For this review, take the finished solid that the model builds, in its own axes (mm). Face numbers are marked on the shaded views. A direction names the side the tool comes from. Round coordinates to 2 decimals unless told otherwise and drop trailing zeros. Loops run counter-clockwise (first coordinate to the right, second up) from the corner with the lowest first, then second, coordinate; pieces in that order, holes last. Notation, with made-up numbers: (-9, 55.5) -> (18, 55.5) arc R20 cw to (18, 86.5) -> close; hole circle Ø7 at (-32.5, -5.5). An arc over 180 degrees is marked (long way). Write each question's results on one line, items separated by ' | '.
```python
from build123d import *

# Parameters (mm, degrees)
SKETCH1_W           = 25.4
SKETCH1_H           = 25.4
BOSS_EXTRUDE1_DEPTH = 1.5875
BOSS_EXTRUDE2_DEPTH = 3.302


with BuildPart() as part:
    # Sketch1 → Boss-Extrude1 (new body)
    with BuildSketch(Plane(origin=(0, 0, 0), x_dir=(1, 0, 0), z_dir=(0, 1, 0))):
        with Locations((-11.947275054, 12.711155892)):
            Rectangle(SKETCH1_W, SKETCH1_H)
    extrude(amount=BOSS_EXTRUDE1_DEPTH)

    # Sketch2 → Boss-Extrude2 (add)
    with BuildSketch(Plane(origin=(0, 0, 0), x_dir=(-1, 0, 0), z_dir=(0, -1, 0))):
        Polygon((17.95497638, 12.711155892), (5.939573728, 12.711155892), (4.886075054, 15.759155892), (4.886075054, 25.411155892), (19.008475054, 25.411155892), (19.008475054, 15.759155892), align=None)
    extrude(amount=BOSS_EXTRUDE2_DEPTH)


solid = part.part
```
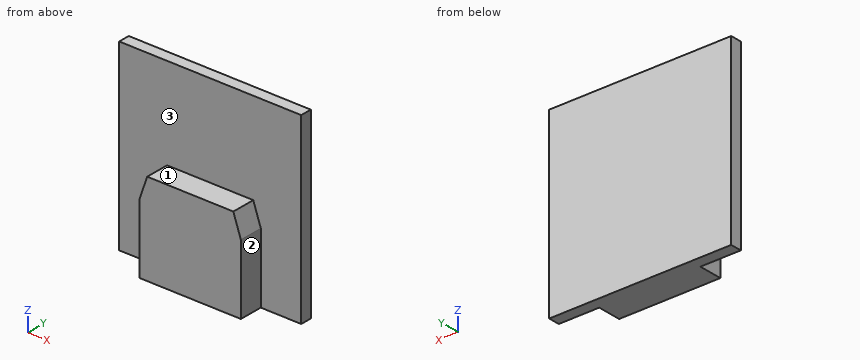
1. To check wall thickness, follow probe 1 along Y at (x, z) = (-2, -20.25); probe 2 along Z at (x, y) = (-6.25, -1.4); probe 3 along X at (y, z) = (-2.75, -22.25). State the ranges of each line that lie inside material, in increasing order.
Values found:
probe 1: y = 0 to 1.59 | probe 2: z = -25.41 to -12.71 | probe 3: x = -19.01 to -4.89
2. Consider section B-B (x = -12.5). State the section outline as (y, z) points, plus the area to 3 significant figures.
Values found:
outline: (-3.3, -25.41) -> (1.59, -25.41) -> (1.59, -0.01) -> (0, -0.01) -> (0, -12.71) -> (-3.3, -12.71) -> close | area: 82.3 mm2
3. Tool access review of the marked faces 1, 2 and 3: name each direction out of +Z, -Z, +X, -X, +Y, -Y from which nothing blocks a thin tool from reaching the whole face with its end or side.
Values found:
face 1: +Z, +X, -X, -Y | face 2: +Z, -Z, +X, -Y | face 3: +Z, -Y
4. Consider section A-A (z = -14.75). State the section outline as (x, y) points, plus the area to 3 significant figures.
Values found:
outline: (-24.65, 0) -> (-18.66, 0) -> (-18.66, -3.3) -> (-5.23, -3.3) -> (-5.23, 0) -> (0.75, 0) -> (0.75, 1.59) -> (-24.65, 1.59) -> close | area: 84.7 mm2
5. Consider section D-D (z = -12). State the section outline as (x, y) points, plus the area to 3 significant figures.
Values found:
outline: (-24.65, 0) -> (0.75, 0) -> (0.75, 1.59) -> (-24.65, 1.59) -> close | area: 40.3 mm2
6. For pin 1 (2 mm diameter, centred on x = -20.5, z = -5, fed in from -Y); pin 2 (1.7 mm diameter, centred on y = -1.5, z = -22.5, fed in from +X); pin 3 (1 mm diameter, centred on x = -12, y = -2.5, fed in from +Z), all flat-tipped, find the tip position at first contact; note any pin that passes through.
Values found:
pin 1: stops at y = 0 | pin 2: stops at x = -4.89 | pin 3: stops at z = -12.71
7. Consider section C-C (y = -2.1). State the section outline as (x, z) points.
Values found:
outline: (-19.01, -25.41) -> (-4.89, -25.41) -> (-4.89, -15.76) -> (-5.94, -12.71) -> (-17.95, -12.71) -> (-19.01, -15.76) -> close
